Print and shaded views of the part. All mm, measured from the part's lowest x, y and z. A direction names the side the tool comes from. Coordinates: 2 decimals unless noted, no trailing zeros. Loops run counter-clockwise (first coordinate to the right, second up) from the corner with the lowest first, then second, coordinate; pieces in that order, holes last. Notation, with made-up numbers: (-7, 34) -> (41, 34) arc R18 cw to (41, 52) -> close; hole circle Ø1 at (-25, 34). An arc over 180 degrees is marked (long way). One line per item, written item: value. Start each with the question number.
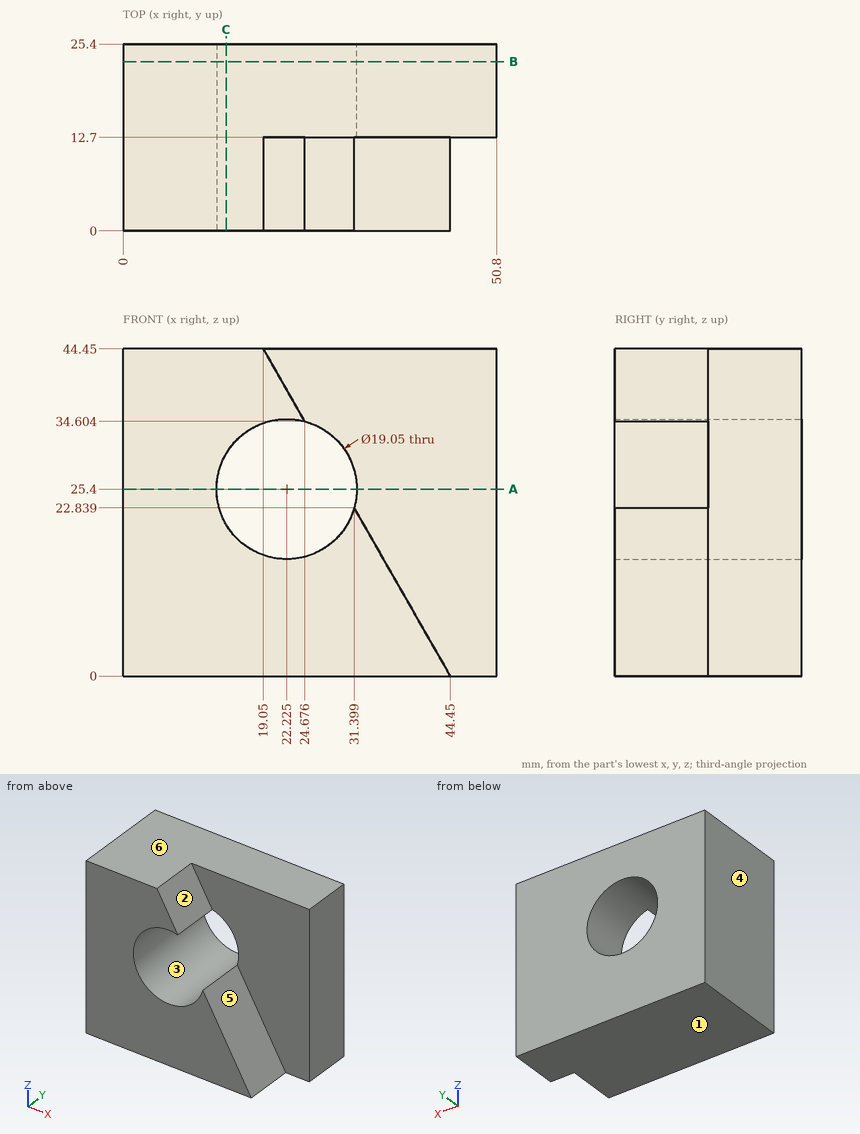
1) Slice it at C-C (x = 14). Give the cut face in (y, z).
2) Probe line 1 (X direction, y = 18.25, z = 25.4); line 2 (Y direction, x = 46.5, z = 12.5); line 3 (Z direction, x = 22, y = 7.5). List the from-to ranges inside material, lowest first. Write a range as from..to.
3) Pull direction X, two halves, no side cores. Call the marked faces 1, 2, 3 and 4: +X half, -X half, draft (parallel to the pull), parting line (faces both ways), or undercut.
4) Slice it at A-A (z = 25.4). Give the cut face in (x, y).
5) Tool access for the marked faces 5 and 6: list every direction of +Z, -Z, +X, -X, +Y, -Y with a clear straight run to the whole face (end or side of a thin tool).
6) Pin check, flat tips, straight feed: pin 1 Ø15 at (x, z) = (22.225, 25.4) entering from +Y; pin 2 Ø16 at (x, z) = (30, 26) entering from -Y; pin 3 Ø1.5 at (x, z) = (45, 16.5) entering from -Y. Stop position of each tip, or through.
7) Slice it at B-B (y = 23). Give the cut face in (x, z) (3 decimals), then the cut area to 3 significant figures.
Check sheet entries:
1. outline: (0, 0) -> (25.4, 0) -> (25.4, 20.6) -> (0, 20.6) -> close; (0, 30.2) -> (25.4, 30.2) -> (25.4, 44.45) -> (0, 44.45) -> close
2. line 1: x = 0..12.7, 31.75..50.8
2. line 2: y = 12.7..25.4
2. line 3: z = 0..15.88, 34.92..39.29
3. face 1: draft
3. face 2: +X half
3. face 3: undercut
3. face 4: -X half
4. outline: (0, 0) -> (12.7, 0) -> (12.7, 25.4) -> (0, 25.4) -> close; (31.75, 12.7) -> (50.8, 12.7) -> (50.8, 25.4) -> (31.75, 25.4) -> close
5. face 5: +Z, +X, -Y
5. face 6: +Z, +X, -X, +Y, -Y
6. pin 1: passes through
6. pin 2: stops at y = 0
6. pin 3: stops at y = 12.7
7. outline: (0, 0) -> (50.8, 0) -> (50.8, 44.45) -> (0, 44.45) -> close; hole circle Ø19.05 at (22.225, 25.4)
7. area: 1,970 mm^2
